Autodesk Inventor part; units mm, degrees
ref_plane "YZ Plane" through (0, 0, 0) normal (1, 0, 0) x (0, 1, 0)
ref_plane "XZ Plane" through (0, 0, 0) normal (0, 1, 0) x (-1, 0, 0)
ref_plane "XY Plane" through (0, 0, 0) normal (0, 0, 1) x (1, 0, 0)
sketch "Sketch1" plane through (0, 0, 0) normal (1, 0, 0) x (0, 1, 0)
  line L0 (0, 0) -> (15.24, 0)
  line L1 (15.24, 0) -> (15.24, -20.32)
  line L2 (15.24, -20.32) -> (0, -20.32)
  line L3 (0, -20.32) -> (0, 0)
  dimension "d0" = 15.24
  dimension "d1" = 20.32
extrude "Extrusion1" add sketch "Sketch1" along normal blind 3.81
sketch "Sketch2" plane through (0, 0, 0) normal (0, 0, 1) x (1, 0, 0)
  line L0 (3.81, 15.24) -> (8.89, 15.24)
  line L1 (8.89, 15.24) -> (14.89, 15.24)
  line L2 (14.89, 15.24) -> (14.89, 10.16)
  line L3 (14.89, 10.16) -> (3.81, 10.16)
  line L4 (3.81, 15.24) -> (3.81, 0)
  line L5 (8.89, 12.9701) -> (11.89, 12.9701)
  line L6 (11.89, 12.9701) -> (11.89, 11.9701)
  line L7 (11.89, 11.9701) -> (5.89, 11.9701)
  line L8 (5.89, 11.9701) -> (5.89, 12.9701)
  line L9 (5.89, 12.9701) -> (5.89, 13.9701)
  line L10 (5.89, 13.9701) -> (11.89, 13.9701)
  line L11 (11.89, 13.9701) -> (11.89, 12.9701)
  line L12 (3.81, 15.24) -> (3.81, 10.16)
  line L13 (0, 12.9701) -> (3.81, 12.9701)
  line L14 (5.89, 12.9701) -> (8.89, 12.9701)
  point P0 (0, 0)
  point P1 (0, 15.24)
  dimension "d4" = 8.89
  dimension "d5" = 6
  dimension "d6" = 5.08
  dimension "d7" = 8.89
  dimension "d8" = 3
  dimension "d9" = 1
  dimension "d10" = 6
  dimension "d11" = 1
extrude "Extrusion2" add sketch "Sketch2" against normal blind 20.32
sketch "Sketch3" plane through (5.89, 11.9701, 0) normal (0, 1, 0) x (1, 0, 0)
  line L0 (0, 0) -> (0, 5.08)
  line L1 (0, 0) -> (0, 20.32)
  line L2 (0, 5.08) -> (2.9845, 5.08)
  line L3 (6, 0) -> (6, 20.32)
  circle A0 centre (2.9845, 5.08) radius 1.27
  line L4 (-2.08, 0) -> (-2.08, 10.16)
  line L5 (-2.08, 0) -> (-2.08, 20.32)
  line L6 (-2.08, 10.16) -> (2.0052, 10.16)
  circle A1 centre (2.9845, 15.24) radius 1.27
  point P0 (-5.89, 0)
  dimension "d14" = 5.08
  dimension "d15" = 2.9845
  dimension "d16" = 2.54
  dimension "d17" = 10.16
extrude "Extrusion3" cut sketch "Sketch3" along normal mid plane 20.32
sketch "Sketch4" plane through (3.81, 0, 0) normal (1, 0, 0) x (0, 0, -1)
  line L0 (0, 0) -> (0, 6.35)
  line L1 (0, 10.16) -> (0, 0)
  line L2 (0, 6.35) -> (5.08, 6.35)
  circle A0 centre (5.08, 6.35) radius 1.905
  line L3 (0, 0) -> (10.16, 0)
  line L4 (0, 0) -> (20.32, 0)
  line L5 (10.16, 0) -> (10.16, 4.445)
  circle A1 centre (15.24, 6.35) radius 1.905
  dimension "d20" = 6.35
  dimension "d21" = 5.08
  dimension "d22" = 3.81
  dimension "d23" = 10.16
extrude "Extrusion4" cut sketch "Sketch4" against normal blind 20.32
fillet "Fillet1" radius 1.5875 1 edges at (3.81, 10.16, -10.16)
properties part number "ExtruderTimingBeltHolder"
Can you work these out from the model? Positions are in its coordinate system, mm. A direction names the side the tool comes from. Round coordinates to 2 decimals unless told otherwise and drop trailing zeros. Loops run counter-clockwise (first coordinate to the right, second up) from the corner with the lowest first, then second, coordinate; pieces in that order, holes last. Notation, with made-up numbers: M -25,42 L -8,42 A35 cw -8,75 Z; hole C 33,72.25 d11. An arc over 180 degrees is marked long. Answer in a Markdown table with one row per item.
1. If we section it at D-D, the plane y = 13.25: Please give me the cut outline in (x, z).
Established:
| item | result |
|---|---|
| outline | M 0,-20.32 L 5.89,-20.32 L 5.89,0 L 0,0 Z; M 11.89,-20.32 L 14.89,-20.32 L 14.89,0 L 11.89,0 Z |
2. I'm going to push flat-ended pins straight in: pin 1 Ø5 at (y, z) = (6.35, -15.24) entering from +X; pin 2 Ø6.5 at (x, z) = (8.5, -12) entering from -Y. Where does each tip first touch, or does it pass through?
Established:
| item | result |
|---|---|
| pin 1 | x = 3.83 |
| pin 2 | y = 10.15 |
3. Please list where these lines run through material, in increasing order: line 1 (X direction, y = 11.6, z = -5.08); line 2 (Y direction, x = 8.75, z = -10); line 3 (Y direction, x = 2.3, z = -15.24) (3 decimals). Write a range as from..to.
Established:
| item | result |
|---|---|
| line 1 | 0..7.6, 10.14..14.89 |
| line 2 | 10.16..11.97, 13.97..15.24 |
| line 3 | 0..4.445, 8.255..15.24 |
4. If we section it at A-A, the plane x = 10.5: Please give me the cut outline in (y, z), plus the area to 3 significant figures.
Established:
| item | result |
|---|---|
| outline | M 10.16,-20.32 L 11.97,-20.32 L 11.97,0 L 10.16,0 Z; M 13.97,-20.32 L 15.24,-20.32 L 15.24,0 L 13.97,0 Z |
| area | 62.6 mm² |
5. Thinking about a two-plate mould opening in X: for faces 4 (the face through (1.932, 6.434, -13.337)), 5 (the face through (8.71, 11.08, -16.5)), 6 (the face through (4.26, 9.68, -10.3)), which applies, pulls with the +X half, pulls with the -X half, needs draft (parallel to the pull), parting line crosses it, or undercut?
Established:
| item | result |
|---|---|
| face 4 | needs draft |
| face 5 | undercut |
| face 6 | pulls with the +X half |
6. If we section it at B-B, the plane y = 6.35: Please give me the cut outline in (x, z) (3 decimals).
Established:
| item | result |
|---|---|
| outline | M 0,-20.32 L 3.81,-20.32 L 3.81,-17.145 L 0,-17.145 Z; M 0,-13.335 L 3.81,-13.335 L 3.81,-6.985 L 0,-6.985 Z; M 0,-3.175 L 3.81,-3.175 L 3.81,0 L 0,0 Z |
7. If we section it at C-C, the plane z = -5.08: Give the number of separate pieces and of enclosed holes in the cut face, plus the area to 3 significant figures.
Established:
| item | result |
|---|---|
| separate pieces | 3 |
| enclosed holes | 0 |
| area | 80.6 mm² |
8. On a 3-axis mill with a long thin cutter (end or side, diameter ignored), from which of +Z, -Z, +X, -X, +Y, -Y can I reach the whole of each face in a straight line? I mean faces 1 (the face through (8.71, 14.6, -13.98)), 2 (the face through (5.89, 13, -10)), 3 (the face through (10, 10.16, -10)). Say none if no direction works.
Established:
| item | result |
|---|---|
| face 1 | +Y, -Y |
| face 2 | +Z, -Z |
| face 3 | +Z, -Z, +X, -Y |
